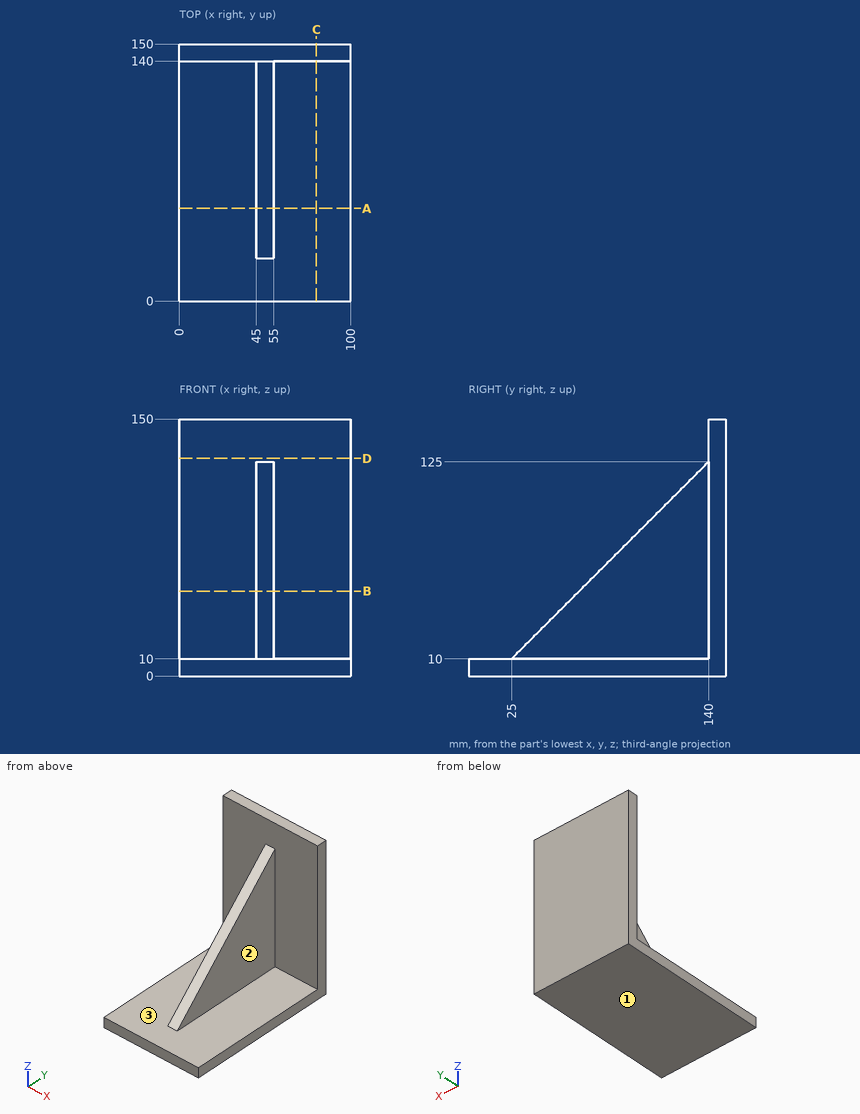
Source: three-view drawing plus pictorial views. Frame: mm from the lowest corner of the part. A direction names the side the tool comes from. Give positions to 0.01 mm unless a question says otherwise; leave off trailing zeros. Loops run counter-clockwise (first coordinate to the right, second up) from the corner with the lowest first, then second, coordinate; pieces in that order, holes last. Notation, with made-up numbers: (21.25, 66) -> (26.25, 66) arc R18 ccw to (26.25, 92) -> close; hole circle Ø1 at (-5, -30). An arc over 180 degrees is marked (long way). Put each result on its own line as item: value. Start each with the question number.
1) Material intervals for probe 1 along Y at (x, z) = (89, 23); probe 2 along Z at (x, y) = (7, 12); probe 3 along X at (y, z) = (111, 49.5), sorted ascending.
2) Cut plane C-C (x = 80). Return loops of the section in (y, z).
3) Cut plane D-D (z = 127). Return loops of the section in (x, y).
4) Contact query for flat-ended pins moving along their axis: P1, Ø8, axis at x = 55, z = 41, coming from the -Y side; P2, Ø5, axis at y = 113, z = 53.5, coming from the +X side; P3, Ø10, axis at x = 40.5, y = 117.5, coming from the +Z side. Output: stop coordinate, or through.
5) Cut plane A-A (y = 54). Return loops of the section in (x, z).
6) Reachability of the marked faces 1, 2 and 3 from +Z, -Z, +X, -X, +Y, -Y: full face, straight path, thin tool, end or side. Return the list, or none.
7) Cut plane B-B (z = 49.5). Return loops of the section in (x, y), then the cut area to 4 significant figures.
Results are:
1. probe 1: y = 140 to 150
1. probe 2: z = 0 to 10
1. probe 3: x = 45 to 55
2. outline: (0, 0) -> (150, 0) -> (150, 150) -> (140, 150) -> (140, 10) -> (0, 10) -> close
3. outline: (0, 140) -> (100, 140) -> (100, 150) -> (0, 150) -> close
4. P1: stops at y = 52
4. P2: stops at x = 55
4. P3: stops at z = 104.68
5. outline: (0, 0) -> (100, 0) -> (100, 10) -> (55, 10) -> (55, 39) -> (45, 39) -> (45, 10) -> (0, 10) -> close
6. face 1: -Z, +X, -X, +Y, -Y
6. face 2: +Z, +X, -Y
6. face 3: +Z, -Y
7. outline: (0, 140) -> (45, 140) -> (45, 64.5) -> (55, 64.5) -> (55, 140) -> (100, 140) -> (100, 150) -> (0, 150) -> close
7. area: 1,755 mm2
